from build123d import *

# Parameters (mm, degrees)
F0_R     = 1.975
F1_DEPTH = 25
F2_R     = 1.49999
F4_DEPTH = 25
F5_DEPTH = 4.8


# Not quite as in the source:
# - a fillet or chamfer is up to 0.001 mm smaller than in the source, because OpenCascade refuses the exact size
# - a feature names something its author has since deleted; it is built from what else it names


with BuildPart() as f1:
    # F0 (on Top) → F1 (new body)
    with BuildSketch(Plane.XY):
        with BuildLine():
            Line((19, 8), (2.6457513111, 8))
            ThreePointArc((2.6457513111, 8), (0, 15), (-2.6457513111, 8))
            Line((-2.6457513111, 8), (-16, 8))
            Line((-16, 8), (-16, 0))
            Line((-16, 0), (19, 0))
            Line((19, 0), (19, 3))
            Line((19, 3), (17.2, 3))
            Line((17.2, 3), (13.5, 3))
            Line((13.5, 3), (-13, 3))
            Line((-13, 3), (-13, 5))
            Line((-13, 5), (19, 5))
            Line((19, 5), (19, 8))
        make_face()
        with Locations((0, 11)):
            Circle(F0_R, mode=Mode.SUBTRACT)
        Polygon((17.2, 3), (19, 3), (19, 4.5), (13.5, 4.5), (13.5, 3), align=None)
    extrude(amount=F1_DEPTH)

    # F2 (radius 1.5 in the source; OpenCascade refuses exactly that, so slightly less here)
    f2_edges = [f1.edges().sort_by_distance(p)[0] for p in [
        (-16, 8, 12.5),
        (-16, 0, 12.5),
        (19, 0, 12.5),
        (19, 5, 12.5),
        (19, 4.5, 12.5),
        (-2.645751, 8, 12.5),
        (19, 8, 12.5),
    ]]
    fillet(f2_edges, radius=F2_R)

    # F3 (on face) → F4 (cut)
    with BuildSketch(Plane.XZ):
        with BuildLine():
            Line((17.50001, 11.6511331714), (17.50001, 13.3488668286))
            ThreePointArc((17.50001, 13.3488668286), (14.2196750343, 12.5), (17.50001, 11.6511331714))
        make_face()
        with BuildLine():
            ThreePointArc((17.7196750343, 12.5), (17.6638689709, 12.9384140794), (17.50001, 13.3488668286))
            Line((17.50001, 13.3488668286), (17.50001, 11.6511331714))
            ThreePointArc((17.50001, 11.6511331714), (17.6638689709, 12.0615859206), (17.7196750343, 12.5))
        make_face()
    extrude(amount=-F4_DEPTH, mode=Mode.SUBTRACT)

    # F3 (on face) → F5 (cut)
    with BuildSketch(Plane.XZ):
        with BuildLine():
            Line((17.50001, 13.3488668286), (17.50001, 13.7876625694))
            ThreePointArc((17.50001, 13.7876625694), (13.9696750343, 12.5), (17.50001, 11.2123374306))
            Line((17.50001, 11.2123374306), (17.50001, 11.6511331714))
            ThreePointArc((17.50001, 11.6511331714), (14.2196750343, 12.5), (17.50001, 13.3488668286))
        make_face()
        with BuildLine():
            ThreePointArc((17.50001, 11.2123374306), (17.8485935971, 11.8146788824), (17.9696750343, 12.5))
            ThreePointArc((17.9696750343, 12.5), (17.8485935971, 13.1853211176), (17.50001, 13.7876625694))
            Line((17.50001, 13.7876625694), (17.50001, 13.3488668286))
            ThreePointArc((17.50001, 13.3488668286), (17.6638689709, 12.9384140794), (17.7196750343, 12.5))
            ThreePointArc((17.7196750343, 12.5), (17.6638689709, 12.0615859206), (17.50001, 11.6511331714))
            Line((17.50001, 11.6511331714), (17.50001, 11.2123374306))
        make_face()
    extrude(amount=-F5_DEPTH, mode=Mode.SUBTRACT)


solid = f1.part
Design review of the part built by this model. Coordinates are the model's own, in mm. A direction names the side the tool comes from. Round coordinates to 2 decimals unless told otherwise and drop trailing zeros. Write each loop counter-clockwise with the first axis right and the second up, starting at its lowest first coordinate (ties: lowest second). Pieces come first, ordered by that corner, then holes. Notation, with made-up numbers: (0, -6.75) -> (30, -6.75) arc R17 ccw to (30, 21.25) -> close; hole circle Ø9 at (51.25, 67). An arc over 180 degrees is marked (long way). One line per item, written item: value. Start each with the question number.
Q1. Add section A-A (x = 0). Give the boundary of the cut face in (y, z) (3 decimals), then the cut area to 3 significant figures.
Q2. The part is to be moulded in two halves that separate along Y. For faces 5 (the face through (1, 6, 0)), 6 (the face through (2, 5, 12)), 7 (the face through (13.8, 4.5, 12.3)), 8 (the face through (-15.57, 0.45, 12.68)), say which applies: pulls with the +Y half, pulls with the -Y half, needs draft (parallel to the pull), parting line crosses it, or undercut.
Q3. Add section B-B (y = 12.5). Give the boundary of the cut face in (x, z).
Q4. Insertion check: P1, Ø4.5, axis at x = -8, z = 17, coming from the +Y side; P2, Ø2.5, axis at x = 0, y = 11, coming from the +Z side; P3, Ø2, axis at y = 11, z = 5, coming from the -X side; P4, Ø3, axis at y = 10, z = 14.5, coming from the -X side. Each pin has a flat end and moves straight along its axis. Give the tip position at first contact, or say it passes through.
Q5. To check wall thickness, follow probe 1 along Y at (x, z) = (-6, 4.5); probe 2 along X at (y, z) = (3.05, 12.5); probe 3 along Y at (x, z) = (0, 19.75) (3 decimals). State the ranges of each line that lie inside material, in increasing order.
Q6. Add section C-C (x = -6). Give the boundary of the cut face in (y, z).
Q7. Tool access review of faces 1 (the face through (18.57, 4.05, 12.68)), 2 (the face through (-10, 8, 12)), 3 (the face through (1, 0, 12)), 4 (the face through (13.5, 4, 12)): name each direction out of +Z, -Z, +X, -X, +Y, -Y from which nothing blocks a thin tool from reaching the whole face with its end or side.
Q8. Add section D-D (y = 1). Give the boundary of the cut face in (x, z).
Response:
1. outline: (0, 0) -> (3, 0) -> (3, 25) -> (0, 25) -> close; (5, 0) -> (9.025, 0) -> (9.025, 25) -> (5, 25) -> close; (12.975, 0) -> (15, 0) -> (15, 25) -> (12.975, 25) -> close
1. area: 226 mm^2
2. face 5: needs draft
2. face 6: undercut
2. face 7: undercut
2. face 8: pulls with the -Y half
3. outline: (-3.71, 0) -> (-1.28, 0) -> (-1.28, 25) -> (-3.71, 25) -> close; (1.28, 0) -> (3.71, 0) -> (3.71, 25) -> (1.28, 25) -> close
4. P1: stops at y = 8
4. P2: passes through
4. P3: stops at x = -4
4. P4: stops at x = -4.17
5. probe 1: y = 0 to 3, 5 to 8
5. probe 2: x = -16 to -13, 13.5 to 13.97, 17.97 to 19
5. probe 3: y = 0 to 3, 5 to 9.025, 12.975 to 15
6. outline: (0, 0) -> (3, 0) -> (3, 25) -> (0, 25) -> close; (5, 0) -> (8, 0) -> (8, 25) -> (5, 25) -> close
7. face 1: +Z, -Z, +X
7. face 2: +Z, -Z, -X, +Y
7. face 3: +Z, -Z, +X, -X, -Y
7. face 4: +Z, -Z
8. outline: (-15.91, 0) -> (18.91, 0) -> (18.91, 25) -> (-15.91, 25) -> close; hole circle Ø4 at (15.97, 12.5)
